Input: part model. Units: mm. Frame: model coordinates. A direction names the side the tool comes from. Coordinates: 2 decimals unless noted, no trailing zeros. Write each loop counter-clockwise with the first axis right and the second up, starting at its lowest first coordinate (ties: lowest second). Pieces come first, ordered by that corner, then holes.
from build123d import *

# Parameters (mm, degrees)
SKETCH1_R           = 1.5
SKETCH1_R_2         = 4
BOSS_EXTRUDE1_DEPTH = 3


with BuildPart() as part:
    # Sketch1 → Boss-Extrude1 (new body)
    with BuildSketch(Plane.XY):
        with BuildLine():
            Line((-49.2, 4.5), (49.2, 4.5))
            ThreePointArc((49.2, 4.5), (49.765685425, 4.734314575), (50, 5.3))
            Line((50, 5.3), (50, 5.2))
            ThreePointArc((50, 5.2), (50.234314575, 5.765685425), (50.8, 6))
            Line((50.8, 6), (70, 6))
            ThreePointArc((70, 6), (72.121320344, 5.121320344), (73, 3))
            Line((73, 3), (73, -3))
            ThreePointArc((73, -3), (72.121320344, -5.121320344), (70, -6))
            Line((70, -6), (50.8, -6))
            ThreePointArc((50.8, -6), (50.234314575, -5.765685425), (50, -5.2))
            Line((50, -5.2), (50, -5.3))
            ThreePointArc((50, -5.3), (49.765685425, -4.734314575), (49.2, -4.5))
            Line((49.2, -4.5), (-49.2, -4.5))
            ThreePointArc((-49.2, -4.5), (-49.765685425, -4.734314575), (-50, -5.3))
            Line((-50, -5.3), (-50, -5.2))
            ThreePointArc((-50, -5.2), (-50.234314575, -5.765685425), (-50.8, -6))
            Line((-50.8, -6), (-70, -6))
            ThreePointArc((-70, -6), (-72.121320344, -5.121320344), (-73, -3))
            Line((-73, -3), (-73, 3))
            ThreePointArc((-73, 3), (-72.121320344, 5.121320344), (-70, 6))
            Line((-70, 6), (-50.8, 6))
            ThreePointArc((-50.8, 6), (-50.234314575, 5.765685425), (-50, 5.2))
            Line((-50, 5.2), (-50, 5.3))
            ThreePointArc((-50, 5.3), (-49.765685425, 4.734314575), (-49.2, 4.5))
        make_face()
        with Locations((-55, 0)):
            Circle(SKETCH1_R, mode=Mode.SUBTRACT)
        with Locations((-67, 0)):
            Circle(SKETCH1_R_2, mode=Mode.SUBTRACT)
        with Locations((67, 0)):
            Circle(SKETCH1_R_2, mode=Mode.SUBTRACT)
        with Locations((55, 0)):
            Circle(SKETCH1_R, mode=Mode.SUBTRACT)
        with BuildLine():
            Line((-46.1, 1.5), (-3.9, 1.5))
            ThreePointArc((-3.9, 1.5), (-2.910050506, 1.089949494), (-2.5, 0.1))
            Line((-2.5, 0.1), (-2.5, -0.1))
            ThreePointArc((-2.5, -0.1), (-2.910050506, -1.089949494), (-3.9, -1.5))
            Line((-3.9, -1.5), (-46.1, -1.5))
            ThreePointArc((-46.1, -1.5), (-47.089949494, -1.089949494), (-47.5, -0.1))
            Line((-47.5, -0.1), (-47.5, 0.1))
            ThreePointArc((-47.5, 0.1), (-47.089949494, 1.089949494), (-46.1, 1.5))
        make_face(mode=Mode.SUBTRACT)
        with BuildLine():
            Line((46.1, 1.5), (3.9, 1.5))
            ThreePointArc((3.9, 1.5), (2.910050506, 1.089949494), (2.5, 0.1))
            Line((2.5, 0.1), (2.5, -0.1))
            ThreePointArc((2.5, -0.1), (2.910050506, -1.089949494), (3.9, -1.5))
            Line((3.9, -1.5), (46.1, -1.5))
            ThreePointArc((46.1, -1.5), (47.089949494, -1.089949494), (47.5, -0.1))
            Line((47.5, -0.1), (47.5, 0.1))
            ThreePointArc((47.5, 0.1), (47.089949494, 1.089949494), (46.1, 1.5))
        make_face(mode=Mode.SUBTRACT)
    extrude(amount=BOSS_EXTRUDE1_DEPTH)


solid = part.part
Item 1: Access query for faces 4 (the face through (1, 0, 3)), 5 (the face through (25, 1.5, 1)). Directions: +Z, -Z, +X, -X, +Y, -Y. A direction counts if a zero-diameter tool reaches every point of the face in a straight line with its end or side. Return the directions, or none.
Item 2: Material intervals for line 1 (Y direction, x = -4, z = 1.6); line 2 (X direction, y = 1.75, z = 0.2); line 3 (Y direction, x = 67, z = 1.2), sorted ascending.
Item 3: Section query C-C, the plane z = 0.6. State how many separate pieces and enclosed holes the cut face has, then the cut area to 3 significant figures.
Item 4: Section query A-A, the plane x = -29.5. Return loops of the section in (y, z).
Item 5: Pin query (flat end, axial travel): pin 1 Ø0.9 at (x, z) = (34, 2) entering from +Y; pin 2 Ø2 at (x, y) = (-35.5, -4) entering from -Z. Return the tip coordinate at first contact, or that it passes through.
Item 6: Section query B-B, the plane x = 67. Return loops of the section in (y, z), then the cut area to 3 significant figures.
Item 7: Pull-direction query (Y, two-part tool) for faces 1 (the face through (1, -4.5, 1)), 2 (the face through (-73, 0, 1)), 3 (the face through (-25, -1.5, 1)); classes: released by +Y, released by -Y, zero draft, split by the parting line, or undercut.
The answers:
1. face 4: +Z, +X, -X, +Y, -Y
1. face 5: +Z, -Z
2. line 1: y = -4.5 to -1.5, 1.5 to 4.5
2. line 2: x = -73 to -70.6, -63.4 to 63.4, 70.6 to 73
2. line 3: y = -6 to -4, 4 to 6
3. separate pieces: 1
3. enclosed holes: 6
3. area: 1,060 mm2
4. outline: (-4.5, 0) - (-1.5, 0) - (-1.5, 3) - (-4.5, 3) - close; (1.5, 0) - (4.5, 0) - (4.5, 3) - (1.5, 3) - close
5. pin 1: stops at y = 4.5
5. pin 2: stops at z = 0
6. outline: (-6, 0) - (-4, 0) - (-4, 3) - (-6, 3) - close; (4, 0) - (6, 0) - (6, 3) - (4, 3) - close
6. area: 12.0 mm2
7. face 1: released by -Y
7. face 2: zero draft
7. face 3: undercut
